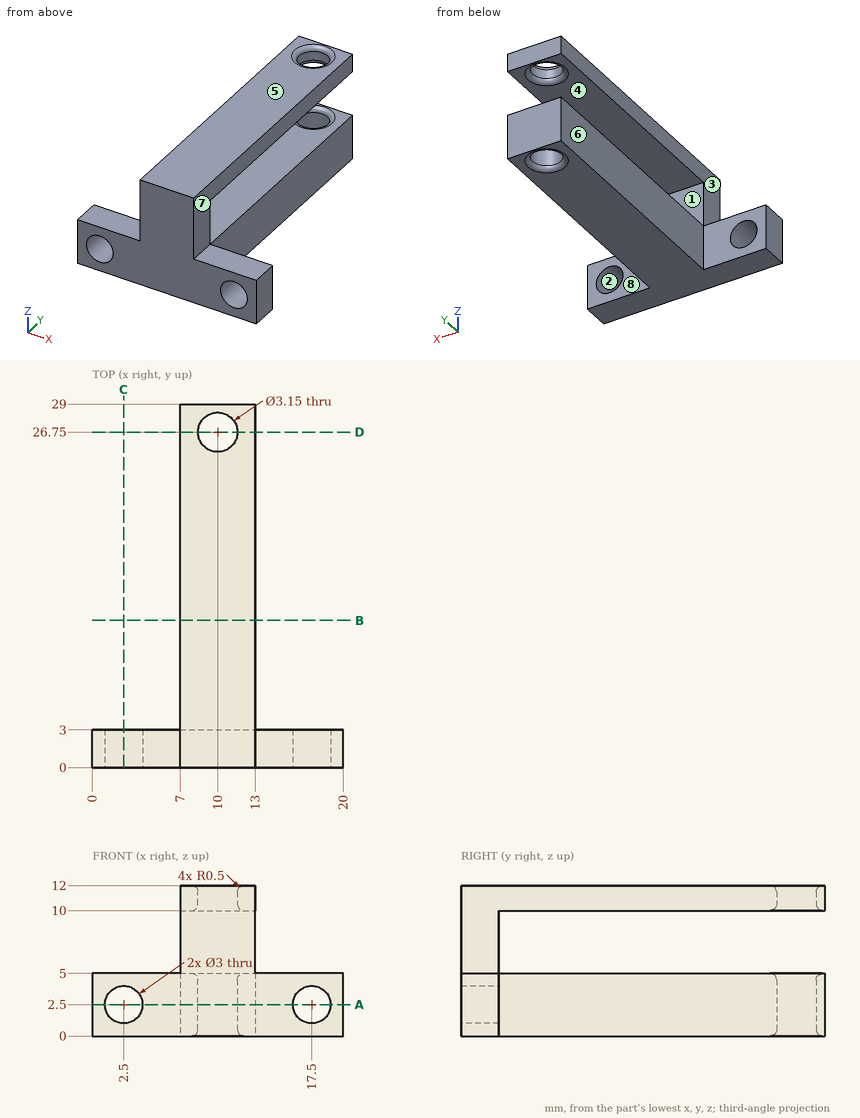
Here's the drawing with two shaded views (mm, measured from the low corner). I have some questions. A direction names the side the tool comes from. Give positions to 0.01 mm unless a question says otherwise; leave off trailing zeros. Loops run counter-clockwise (first coordinate to the right, second up) from the corner with the lowest first, then second, coordinate; pieces in that order, holes last. Notation, with made-up numbers: (-14, 76.25) - (30, 76.25) arc R13 ccw to (30, 101.25) - close; hole circle Ø4 at (-33.75, 48). An arc over 180 degrees is marked (long way). One line per item, written item: value.
(1) I'm going to push flat-ended pins straight in: pin 1 (3.5 mm diameter, centred on x = 15, y = 2, fed in from +Z); pin 2 (2 mm diameter, centred on y = 13.5, z = 9.5, fed in from +X); pin 3 (2 mm diameter, centred on x = 15.5, z = 5, fed in from +Y). Where does each tip first touch, or does it pass through?
Verdict:
pin 1: z = 5
pin 2: x = 13
pin 3: y = 3
(2) If we mould it in two halves opening along X, with no side actions, what happens to the marked faces 1, 2 and 3? For each: released by +X, released by -X, zero draft, split by the parting line, or undercut.
Verdict:
face 1: zero draft
face 2: undercut
face 3: released by -X
(3) I need wall thicknesses on line 1 along X through (y, z) = (1.15, 2.5); line 2 along Z through (x, y) = (12.25, 14); line 3 along Y through (x, z) = (10, 1.55) (3 decimals). Which ranges of each line are inside material? Lowest first, please.
Verdict:
line 1: 0 to 1, 4 to 16, 19 to 20
line 2: 0 to 5, 10 to 12
line 3: 0 to 25.175, 28.325 to 29
(4) If we section it at D-D, the plane y = 26.75: List the corners of the cut face in (x, z) for me (3 decimals), plus the area to 3 significant figures.
Verdict:
outline: (7, 0) - (7.925, 0) arc R0.5 ccw to (8.425, 0.5) - (8.425, 4.5) arc R0.5 ccw to (7.925, 5) - (7, 5) - close; (7, 10) - (7.925, 10) arc R0.5 ccw to (8.425, 10.5) - (8.425, 11.5) arc R0.5 ccw to (7.925, 12) - (7, 12) - close; (11.575, 0.5) arc R0.5 ccw to (12.075, 0) - (13, 0) - (13, 5) - (12.075, 5) arc R0.5 ccw to (11.575, 4.5) - close; (11.575, 10.5) arc R0.5 ccw to (12.075, 10) - (13, 10) - (13, 12) - (12.075, 12) arc R0.5 ccw to (11.575, 11.5) - close
area: 19.5 mm^2
(5) On a 3-axis mill with a long thin cutter (end or side, diameter ignored), from which of +Z, -Z, +X, -X, +Y, -Y can I reach the whole of each face in a straight line? I mean the marked faces 4, 5, 6, 7 and 8. Say none if no direction works.
Verdict:
face 4: +X, -X, +Y
face 5: +Z, +X, -X, +Y, -Y
face 6: +Z, -Z, -X, +Y
face 7: +Z, +X, +Y, -Y
face 8: +Z, -Z, +X, +Y
(6) If we section it at C-C, the plane x = 2.5: List the corners of the cut face in (y, z) for me, plus the area to 3 significant figures.
Verdict:
outline: (0, 0) - (3, 0) - (3, 1) - (0, 1) - close; (0, 4) - (3, 4) - (3, 5) - (0, 5) - close
area: 6.00 mm^2
(7) If we section it at A-A, the plane z = 2.5: List the corners of the cut face in (x, y) for me (3 decimals).
Verdict:
outline: (0, 0) - (1, 0) - (1, 3) - (0, 3) - close; (4, 0) - (16, 0) - (16, 3) - (13, 3) - (13, 29) - (7, 29) - (7, 3) - (4, 3) - close; (19, 0) - (20, 0) - (20, 3) - (19, 3) - close; hole circle Ø3.15 at (10, 26.75)
(8) If we section it at B-B, the plane y = 11.75: List the corners of the cut face in (x, z) for me.
Verdict:
outline: (7, 0) - (13, 0) - (13, 5) - (7, 5) - close; (7, 10) - (13, 10) - (13, 12) - (7, 12) - close
